Autodesk Inventor part; units mm, degrees
ref_plane "YZ Plane" through (0, 0, 0) normal (1, 0, 0) x (0, 1, 0)
ref_plane "XZ Plane" through (0, 0, 0) normal (0, 1, 0) x (-1, 0, 0)
ref_plane "XY Plane" through (0, 0, 0) normal (0, 0, 1) x (1, 0, 0)
sketch "Sketch1" plane through (0, 0, 0) normal (0, 0, 1) x (1, 0, 0)
  line L0 (-172, 172) -> (172, 172)
  line L1 (172, 172) -> (172, -172)
  line L2 (172, -172) -> (-172, -172)
  line L3 (-172, -172) -> (-172, 172)
  point P0 (0, 0)
  dimension "d0" = 344
  dimension "d1" = 344
  dimension "d2" = 172
  dimension "d3" = 172
extrude "Extrusion1" add sketch "Sketch1" along normal blind 8
sketch "Sketch3" plane through (0, 0, 0) normal (0, 0, -1) x (-1, 0, 0)
  circle A0 centre (-102, 102) radius 53.5
  circle A1 centre (52, -28) radius 53.5
  circle A2 centre (52, -28) radius 12.5 construction
  circle A3 centre (-102, 102) radius 12.5 construction
  point P0 (0, 0)
  dimension "d18" = 107
  dimension "d19" = 107
extrude "Extrusion2" cut sketch "Sketch3" against normal through all
sketch "Sketch4" plane through (0, 0, 0) normal (0, 0, -1) x (-1, 0, 0)
  line L0 (118.61, 61.21) -> (118.61, -90.79)
  line L1 (119.61, -91.79) -> (167.35, -91.79)
  line L2 (168.35, -90.79) -> (168.35, 61.21)
  line L3 (167.35, 62.21) -> (119.61, 62.21)
  line L4 (162, 69.21) -> (63.35, 69.21)
  line L5 (63.35, 106.21) -> (162, 106.21)
  line L6 (63.35, 69.21) -> (63.35, 106.21)
  line L7 (163.35, 69.21) -> (163.35, 106.21)
  arc A0 (118.61, -90.79) -> (119.61, -91.79) centre (119.61, -90.79) ccw
  arc A1 (167.35, -91.79) -> (168.35, -90.79) centre (167.35, -90.79) ccw
  arc A2 (168.35, 61.21) -> (167.35, 62.21) centre (167.35, 61.21) ccw
  arc A3 (119.61, 62.21) -> (118.61, 61.21) centre (119.61, 61.21) ccw
  line L8 (162, 69.21) -> (163.35, 69.21)
  line L9 (163.35, 106.21) -> (162, 106.21)
  point P0 (0, 0)
extrude "Extrusion3" cut sketch "Sketch4" against normal through all
sketch "Sketch5" plane through (0, 0, 0) normal (0, 0, -1) x (-1, 0, 0)
  line L0 (-87, -15) -> (-87, -163) construction
  line L1 (-171, -15) -> (-87, -15) construction
  line L2 (-171, -163) -> (-171, -15) construction
  line L3 (-87, -163) -> (-171, -163) construction
  line L4 (-91, -154) -> (-91, -24)
  line L5 (-96, -19) -> (-162, -19)
  line L6 (-167, -24) -> (-167, -154)
  line L7 (-162, -159) -> (-96, -159)
  arc A0 (-96, -159) -> (-91, -154) centre (-96, -154) ccw
  arc A1 (-167, -154) -> (-162, -159) centre (-162, -154) ccw
  arc A2 (-162, -19) -> (-167, -24) centre (-162, -24) ccw
  arc A3 (-91, -24) -> (-96, -19) centre (-96, -24) ccw
  point P0 (0, 0)
  dimension "d20" = 4
  dimension "d21" = 5
extrude "Extrusion4" cut sketch "Sketch5" against normal through all
equation "\"d0\" = edge_length - 2 * wall_width"
equation "\"d1\" = edge_length - 2 * wall_width"
equation "\"d4\" = wall_width_small"
properties part number "Element"
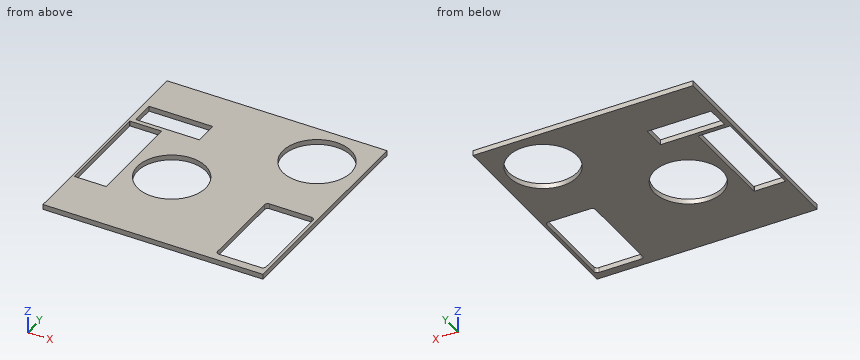
Geometry check sheet. Reference: the model listing, model coordinates, mm. Round coordinates to 2 decimals unless told otherwise and drop trailing zeros. Write each loop counter-clockwise with the first axis right and the second up, starting at its lowest first coordinate (ties: lowest second). Pieces come first, ordered by that corner, then holes. Notation, with made-up numbers: (15, 57.5) -> (41, 57.5) arc R7 ccw to (41, 68.5) -> close; hole circle Ø5 at (23, 15.25). An arc over 180 degrees is marked (long way). One line per item, written item: value. Start each with the question number.
(1) Cross-section at B-B, the plane x = 102. Record the cut outline in (y, z), and give its area (3 significant figures).
(2) Cross-section at A-A, the plane y = 41. Record the cut outline in (x, z), and give its area (3 significant figures).
(3) Cross-section at D-D, the plane y = -28. Record the cut outline in (x, z), and give its area (3 significant figures).
(4) Scan lines: line 1 (X direction, y = -83, z = 0.5); line 2 (Y direction, x = -134, z = 4); line 3 (Y direction, x = 102, z = 1.5). Record each from-to range of solid material in increasing order. Write a range as [from, to].
(5) Cross-section at C-C, the plane z = 4. Record the cut outline in (x, y).
Answer:
1. outline: (-172, 0) -> (-159, 0) -> (-159, 8) -> (-172, 8) -> close; (-19, 0) -> (48.5, 0) -> (48.5, 8) -> (-19, 8) -> close; (155.5, 0) -> (172, 0) -> (172, 8) -> (155.5, 8) -> close
1. area: 776 mm²
2. outline: (-172, 0) -> (-168.35, 0) -> (-168.35, 8) -> (-172, 8) -> close; (-118.61, 0) -> (172, 0) -> (172, 8) -> (-118.61, 8) -> close
2. area: 2,350 mm²
3. outline: (-172, 0) -> (-168.35, 0) -> (-168.35, 8) -> (-172, 8) -> close; (-118.61, 0) -> (-105.5, 0) -> (-105.5, 8) -> (-118.61, 8) -> close; (1.5, 0) -> (91, 0) -> (91, 8) -> (1.5, 8) -> close; (167, 0) -> (172, 0) -> (172, 8) -> (167, 8) -> close
3. area: 890 mm²
4. line 1: [-172, -168.35], [-118.61, 91], [167, 172]
4. line 2: [-172, -91.79], [62.21, 69.21], [106.21, 172]
4. line 3: [-172, -159], [-19, 48.5], [155.5, 172]
5. outline: (-172, -172) -> (172, -172) -> (172, 172) -> (-172, 172) -> close; hole (-168.35, -90.79) arc R1 ccw to (-167.35, -91.79) -> (-119.61, -91.79) arc R1 ccw to (-118.61, -90.79) -> (-118.61, 61.21) arc R1 ccw to (-119.61, 62.21) -> (-167.35, 62.21) arc R1 ccw to (-168.35, 61.21) -> close; hole (-163.35, 69.21) -> (-63.35, 69.21) -> (-63.35, 106.21) -> (-163.35, 106.21) -> close; hole circle Ø107 at (-52, -28); hole circle Ø107 at (102, 102); hole (91, -154) arc R5 ccw to (96, -159) -> (162, -159) arc R5 ccw to (167, -154) -> (167, -24) arc R5 ccw to (162, -19) -> (96, -19) arc R5 ccw to (91, -24) -> close
